Build history of the part. All positions in model axes, mm. A direction names the side the tool comes from. Coordinates: 2 decimals unless noted, no trailing zeros. Loops run counter-clockwise (first coordinate to the right, second up) from the corner with the lowest first, then second, coordinate; pieces in that order, holes last.
(1) Tool access for faces 4 (the face through (19, 120.65, -3)), 5 (the face through (19, 6.35, -19)), 6 (the face through (19, 57.15, -35)), 7 (the face through (1.449, 9.658, -36.572)): list every direction of +Z, -Z, +X, -X, +Y, -Y with a clear straight run to the whole face (end or side of a thin tool).
(2) Slice it at C-C (z = -19.05). Give the cut face in (x, y), and give its area (3 significant figures).
(3) Slice it at D-D (x = 24.5). Give the cut face in (y, z), and give its area (3 significant figures).
(4) Two-plate mould, pull along X, no slides. Class faces 1 (the face through (17.88, 3.131, -17.977)), 2 (the face through (36.651, 9.658, -36.572)), 3 (the face through (19, 146.05, -10)): pulls with the +X half, pulls with the -X half, needs draft (parallel to the pull), parting line crosses it, or undercut.
(5) Wall check: L1, parallel to X at y = 3, z = -19; L2, parallel to Z at x = 19.05, y = 2.75; L3, parallel to Y at x = 8, z = -1.5. Give the ranges that are in metal, low to high.
(6) Slice it at B-B (y = 22.5). Give the cut face in (x, z).
(7) Slice it at A-A (x = 19.05). Give the cut face in (y, z), and give its area (3 significant figures).
(8) Flat gauge pins, fed straight in: P1, Ø8, axis at x = 24, y = 52, coming from the -Z side; P2, Ø5, axis at x = 28, z = -2.5, coming from the +Y side; P3, Ø2.5, axis at x = 19, z = -19, coming from the -Y side. Where does each tip first touch, or does it go through?
from build123d import *

# Parameters (mm, degrees)
F1_DEPTH = 38.1
F2_R     = 1.5875
F3_DEPTH = 6.35
F4_R     = 5.08


with BuildPart() as f1:
    # F0 (on Right) → F1 (new body)
    with BuildSketch(Plane.YZ):
        Polygon((120.65, 0), (0, 0), (0, -38.1), (19.05, -38.1), (19.05, -31.75), (57.15, -31.75), (57.15, -38.1), (69.85, -38.1), (146.05, -12.7), (146.05, -6.35), (120.65, -6.35), align=None)
    extrude(amount=F1_DEPTH)

    # F2 (on face) → F3 (cut)
    with BuildSketch(Plane.XZ):
        with Locations((19.05, -19.05)):
            Circle(F2_R)
    extrude(amount=-F3_DEPTH, mode=Mode.SUBTRACT)

    # F4
    f4_edges = [f1.edges().sort_by_distance(p)[0] for p in [
        (38.1, 60.325, 0),
        (0, 60.325, 0),
        (38.1, 9.525, -38.1),
        (0, 9.525, -38.1),
    ]]
    fillet(f4_edges, radius=F4_R)


solid = f1.part
Response values:
1. face 4: +Z, +X, -X, +Y
1. face 5: -Y
1. face 6: -Z, +X, -X
1. face 7: -Z, -X, -Y
2. outline: (0, 0) - (17.46, 0) - (17.46, 6.35) - (20.64, 6.35) - (20.64, 0) - (38.1, 0) - (38.1, 127) - (0, 127) - close
2. area: 4,820 mm2
3. outline: (0, -38.1) - (19.05, -38.1) - (19.05, -31.75) - (57.15, -31.75) - (57.15, -38.1) - (69.85, -38.1) - (146.05, -12.7) - (146.05, -6.35) - (120.65, -6.35) - (120.65, 0) - (0, 0) - close
3. area: 4,190 mm2
4. face 1: undercut
4. face 2: pulls with the +X half
4. face 3: needs draft
5. L1: x = 0 to 17.46, 20.64 to 38.1
5. L2: z = -38.1 to -20.64, -17.46 to 0
5. L3: y = 0 to 120.65
6. outline: (0, -31.75) - (38.1, -31.75) - (38.1, -5.08) arc R5.08 ccw to (33.02, 0) - (5.08, 0) arc R5.08 ccw to (0, -5.08) - close
7. outline: (0, -38.1) - (19.05, -38.1) - (19.05, -31.75) - (57.15, -31.75) - (57.15, -38.1) - (69.85, -38.1) - (146.05, -12.7) - (146.05, -6.35) - (120.65, -6.35) - (120.65, 0) - (0, 0) - (0, -17.46) - (6.35, -17.46) - (6.35, -20.64) - (0, -20.64) - close
7. area: 4,170 mm2
8. P1: stops at z = -31.75
8. P2: stops at y = 120.65
8. P3: stops at y = 6.35
